The listing builds one solid part. Answer for the finished solid, in the listing's coordinates (mm). Face numbers are marked on the shaded views. Round coordinates to 2 decimals unless told otherwise and drop trailing zeros. Write each loop counter-clockwise with the first axis right and the second up, starting at its lowest first coordinate (ties: lowest second). Pieces come first, ordered by that corner, then holes.
Item 1: For a pull along Y with two mould halves and no side action, classify the marked faces 1, 2 and 3 as +Y half, -Y half, draft (parallel to the pull), parting line (faces both ways), or undercut.
Item 2: Find section D-D on y = 18. Give the vertices of the cut face in (x, z) (3 decimals), then the cut area to 3 significant figures.
Item 3: Each of these flat-tipped pins is pushed along its axis until it touches: pin 1 (1.3 mm diameter, centred on x = 31.5, z = -1.5, fed in from -Y); pin 2 (2 mm diameter, centred on y = 15, z = 0, fed in from -X) (3 decimals); pin 3 (5 mm diameter, centred on x = -15.5, y = 16.5, fed in from -Z). Where does it stop, or does it pass through?
Item 4: Find the intervals of material crossed by probe 1 along Y at (x, z) = (-23.5, -0.9); probe 2 along X at (y, z) = (10, 0.85) (3 decimals); probe 3 along Y at (x, z) = (-33, 0), in increasing order.
Item 5: Find section B-B on x = -21.5. Give the vertices of the cut face in (y, z).
Item 6: Find section A-A on y = 21.25. Give the vertices of the cut face in (x, z) (3 decimals).
Item 7: Find section C-C on z = -1.5. Give the vertices of the cut face in (x, y) (3 decimals), then the cut area to 3 significant figures.
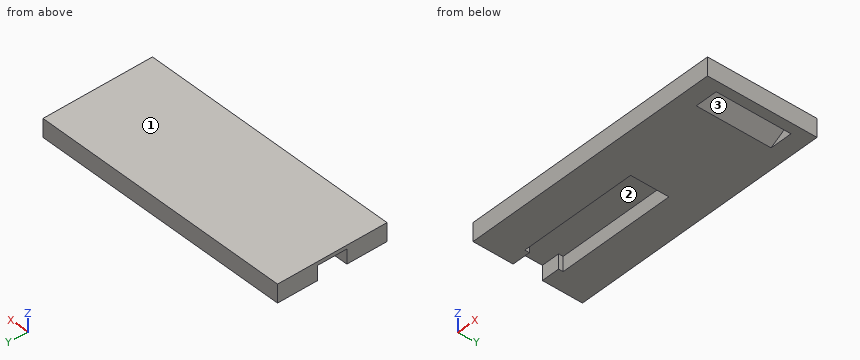
```python
from build123d import *

# Parameters (mm, degrees)
SKETCH_1_W          = 72.07
SKETCH_1_H          = 5
EXTRUDE_1_DEPTH     = 30
CUT_EXTRUDE_1_DEPTH = 4
CUT_EXTRUDE_START   = -15
CUT_EXTRUDE_2_DEPTH = 10.25


with BuildPart() as part:
    # 草圖1 → 填料-伸長1 (new body)
    with BuildSketch(Plane(origin=(0, 0, 0), x_dir=(1, 0, 0), z_dir=(0, 1, 0))):
        Rectangle(SKETCH_1_W, SKETCH_1_H)
    extrude(amount=EXTRUDE_1_DEPTH)

    # 草圖2 → 除料-伸長1 (cut)
    with BuildSketch(Plane(origin=(0, 0, -2.5), x_dir=(-1, 0, 0), z_dir=(0, 0, -1))):
        Polygon((36.035, 19), (36.035, 11), (31.035, 11), (31.035, 9.75), (-1.465, 9.75), (-1.465, 20.25), (31.035, 20.25), (31.035, 19), align=None)
    extrude(amount=-CUT_EXTRUDE_1_DEPTH, mode=Mode.SUBTRACT)

    # 草圖3 → 除料-伸長2 (cut, symmetric)
    with BuildSketch(Plane(origin=(0, 30, 0), x_dir=(1, 0, 0), z_dir=(0, 1, 0)).offset(CUT_EXTRUDE_START)):
        Polygon((33.364978213, 2.5), (31.835, -0.15), (27.24506536, 2.5), align=None)
    extrude(amount=CUT_EXTRUDE_2_DEPTH, both=True, mode=Mode.SUBTRACT)


solid = part.part
```
Check values:
1. face 1: draft
1. face 2: undercut
1. face 3: undercut
2. outline: (-36.035, 1.5) - (1.465, 1.5) - (1.465, -2.5) - (27.245, -2.5) - (31.835, 0.15) - (33.365, -2.5) - (36.035, -2.5) - (36.035, 2.5) - (-36.035, 2.5) - close
2. area: 202 mm2
3. pin 1: stops at y = 0
3. pin 2: stops at x = 1.465
3. pin 3: stops at z = 1.5
4. probe 1: y = 0 to 9.75, 20.25 to 30
4. probe 2: x = -36.035 to -31.035, 1.465 to 36.035
4. probe 3: y = 0 to 11, 19 to 30
5. outline: (0, -2.5) - (9.75, -2.5) - (9.75, 1.5) - (20.25, 1.5) - (20.25, -2.5) - (30, -2.5) - (30, 2.5) - (0, 2.5) - close
6. outline: (-36.035, -2.5) - (27.245, -2.5) - (31.835, 0.15) - (33.365, -2.5) - (36.035, -2.5) - (36.035, 2.5) - (-36.035, 2.5) - close
7. outline: (-36.035, 0) - (36.035, 0) - (36.035, 30) - (-36.035, 30) - (-36.035, 19) - (-31.035, 19) - (-31.035, 20.25) - (1.465, 20.25) - (1.465, 9.75) - (-31.035, 9.75) - (-31.035, 11) - (-36.035, 11) - close; hole (28.977, 4.75) - (32.788, 4.75) - (32.788, 25.25) - (28.977, 25.25) - close
7. area: 1,700 mm2
